Can you work these out from the model? Positions are in its coordinate system, mm. Face numbers are marked on the shaded views. A direction names the side the tool comes from. Coordinates: 2 decimals unless noted, no trailing zeros. Order: outer loops, then holes, each group sorted by start corner. A loop starts at its lowest first (then second) coordinate and runs counter-clockwise, first axis right, second up. Notation, with made-up numbers: (85.25, -17) - (104.25, -17) arc R19 ccw to (104.25, 4) - close; hole circle Ø1 at (74, 18). An arc over 180 degrees is marked (long way). Return JSON: item names as keys, results as strings. Group by question number.
1) Which directions (+Z, -Z, +X, -X, +Y, -Y) give clear straight access to the entire face, cutting with the end or side of a thin tool? Please do the marked faces 1, 2 and 3.
2) If I drill on line 1 along X through (y, z) = (-0.75, 5); line 2 along Z through (x, y) = (13, 7.05); line 3 along Y through (x, z) = (0, 3.85), over which ranges is the centre line in solid material (lowest first)?
3) Imagine slicing it at C-C (x = 0). Write out the boundary of the cut face in (y, z).
4) Imagine slicing it at D-D (y = 5.75). Write out the boundary of the cut face in (x, z).
5) Imagine slicing it at A-A (y = 0). Write out the boundary of the cut face in (x, z).
6) For pin 1 Ø6 at (x, y) = (-4, -1.5) entering from -Z; pin 2 Ø3 at (x, z) = (1, 2) entering from -Y; pin 3 Ø1.5 at (x, y) = (-8, -3.5) entering from +Z; pin 4 Ø2 at (x, z) = (-10.5, 11) entering from +Y, each with a flat end and sliding along its axis, tell me the tip position at first contact or that it passes through.
7) Imagine slicing it at B-B (z = 16). Write out the boundary of the cut face in (x, y).
8) If we mould it in two halves opening along X, with no side actions, what happens to the marked faces 4, 5, 6 and 7? For each: pulls with the +X half, pulls with the -X half, needs draft (parallel to the pull), parting line crosses it, or undercut.
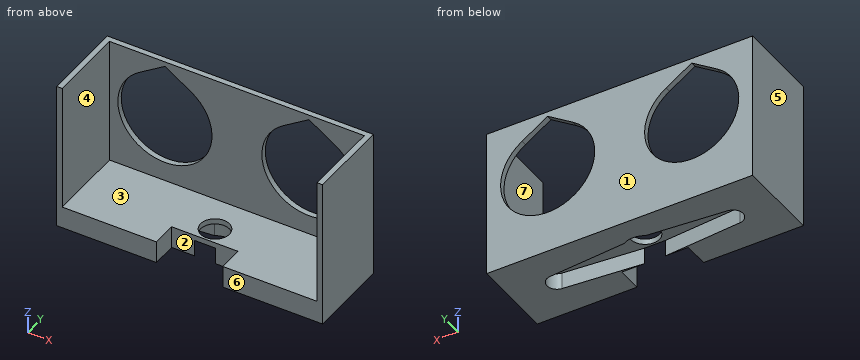
Solid Edge part; units mm, degrees
sketch "Sketch1" plane through (0, 0, 0) normal (0, 0, 1) x (1, 0, 0)
  line L0 (-24, -7.5) -> (24, -7.5)
  line L1 (24, -7.5) -> (24, 7.5)
  line L2 (24, 7.5) -> (-24, 7.5)
  line L3 (-24, 7.5) -> (-24, -7.5)
  dimension "D1" = 24
  dimension "D2" = 24
extrude "Protrusion1" add sketch "Sketch1" along normal blind 5
sketch "Sketch2" plane through (0, 0, 5) normal (0, 0, 1) x (1, 0, 0)
  line L0 (-24, -7.5) -> (24, -7.5)
  line L1 (24, -7.5) -> (24, 7.5)
  line L2 (24, 7.5) -> (-24, 7.5)
  line L3 (-24, 7.5) -> (-24, -7.5)
extrude "ProtrusiónExtruida_5" add sketch "Sketch2" along normal blind 22
shell "Espesor_3" thickness 1 removed faces 2 at (-16.48, -7.5, 22.23) at (-16.48, -4.85, 27)
sketch "Sketch3" plane through (0, -0.5, 1) normal (0, 0, 1) x (1, 0, 0)
  line L0 (-23, -7) -> (-23, 7)
  line L1 (-23, 7) -> (23, 7)
  line L2 (23, 7) -> (23, -7)
  line L3 (23, -7) -> (-23, -7)
extrude "ProtrusiónExtruida_6" add sketch "Sketch3" along normal blind 3
sketch "Sketch4" plane through (0, 0, 0) normal (0, 0, -1) x (1, 0, 0)
  arc A0 (-1.8978, 3.0001) -> (1.8978, 3.0001) centre (0, 0) cw
  line L0 (1.8978, 3.0001) -> (16.0507, 1.7935)
  arc A1 (16.0507, 1.7935) -> (16.0507, -1.7935) centre (15.8978, 0) cw
  line L1 (1.8982, -2.9999) -> (16.0507, -1.7935)
  arc A2 (1.8982, -2.9999) -> (-1.8982, -2.9999) centre (0, 0) cw
  line L2 (-1.8982, -2.9999) -> (-16.0507, -1.7935)
  arc A3 (-16.0507, 1.7935) -> (-16.0507, -1.7935) centre (-15.8978, 0) ccw
  line L3 (-1.8978, 3.0001) -> (-16.0507, 1.7935)
  dimension "D1" = 15.8978
extrude "VaciadoExtruido_1" cut sketch "Sketch4" against normal blind 3
hole "Agujero_2" at (0, 0, 4) direction (0, 0, -1) diameter 2.1 end up to next
sketch "Sketch5" plane through (0, -0.5, 4) normal (0, 0, 1) x (1, 0, 0)
  circle A0 centre (0, 0.5) radius 2.6
extrude "VaciadoExtruido_4" cut sketch "Sketch5" against normal blind 1.4
sketch "Sketch6" plane through (0, -0.5, 4) normal (0, 0, 1) x (1, 0, 0)
  line L0 (-6, -7) -> (-6, -2.5)
  line L1 (-6, -2.5) -> (6, -2.5)
  line L2 (6, -2.5) -> (6, -7)
  line L3 (6, -7) -> (-6, -7)
  dimension "D1" = 6
  dimension "D2" = 6
extrude "Cutout1" cut sketch "Sketch6" against normal up to next
hole "Agujero_3" at (13, 6.5, 16) direction (0, 1, 0) diameter 17 end up to next
hole "Hole1" at (-13, 6.5, 16) direction (0, 1, 0) diameter 17 end up to next
sketch "Sketch7" plane through (0, 7.5, 13.5) normal (0, 1, 0) x (-1, 0, 0)
  line L0 (-13, 12.6313) -> (-8.3746, 9.6313)
  line L1 (-17.6254, 9.6313) -> (-8.3746, 9.6313)
  line L2 (-13, 12.6313) -> (-17.6254, 9.6313)
  line L3 (13, 12.6313) -> (8.3746, 9.6313)
  line L4 (8.3746, 9.6313) -> (17.6254, 9.6313)
  line L5 (17.6254, 9.6313) -> (13, 12.6313)
extrude "Cutout2" cut sketch "Sketch7" against normal up to next
Calculated:
{
 "1": {"face 1": "+Z, -Z, +X, -X, +Y", "face 2": "+Z, -Z, -Y", "face 3": "+Z, -Y"},
 "2": {"line 1": "-24 to -23, 23 to 24", "line 2": "0 to 7.5, 26.13 to 27", "line 3": "-3 to -2.6, 2.6 to 7.5"},
 "3": {"outline": "(-3, 3) - (-2.6, 3) - (-2.6, 4) - (-3, 4) - close; (2.6, 3) - (3.55, 3) - (3.55, 0) - (7.5, 0) - (7.5, 27) - (6.5, 27) - (6.5, 4) - (2.6, 4) - close"},
 "4": {"outline": "(-24, 0) - (24, 0) - (24, 27) - (23, 27) - (23, 4) - (-23, 4) - (-23, 27) - (-24, 27) - close"},
 "5": {"outline": "(-24, 0) - (-17.7, 0) - (-17.7, 3) - (-2.6, 3) - (-2.6, 4) - (-23, 4) - (-23, 27) - (-24, 27) - close; (2.6, 3) - (17.7, 3) - (17.7, 0) - (24, 0) - (24, 27) - (23, 27) - (23, 4) - (2.6, 4) - close"},
 "6": {"pin 1": "z = 0", "pin 2": "y = -3", "pin 3": "z = 4", "pin 4": "through"},
 "7": {"outline": "(-24, -7.5) - (-23, -7.5) - (-23, 6.5) - (-21.5, 6.5) - (-21.5, 7.5) - (-24, 7.5) - close; (-4.5, 6.5) - (4.5, 6.5) - (4.5, 7.5) - (-4.5, 7.5) - close; (21.5, 6.5) - (23, 6.5) - (23, -7.5) - (24, -7.5) - (24, 7.5) - (21.5, 7.5) - close"},
 "8": {"face 4": "undercut", "face 5": "pulls with the -X half", "face 6": "needs draft", "face 7": "undercut"}
}
